Part model, mm, in its own coordinate system. A direction names the side the tool comes from. Give positions to 0.01 mm unless a question says otherwise; leave off trailing zeros. Order: outer loops, then holes, each group sorted by start corner. A loop starts at its lowest first (then second) coordinate and runs counter-clockwise, first axis right, second up. Notation, with made-up numbers: (3.25, -24.75) -> (24.25, -24.75) arc R21 cw to (24.25, 1.25) -> close; hole circle Ø1 at (38.25, 37). An arc over 180 degrees is marked (long way). Write item = value, one per line. Start each with the question number.
Item 1: Flat gauge pins, fed straight in: P1, Ø5, axis at y = -23.5, z = 1.5, coming from the -X side; P2, Ø1.5, axis at x = 15.5, z = 6, coming from the -Y side; P3, Ø1, axis at x = -35, z = 6.5, coming from the +Y side. Where does each tip first touch, or does it go through?
Item 2: Band-saw the part on A-A on x = 0. Write the cut outline in (y, z).
Item 3: Band-saw the part on B-B on y = 0. Write the cut outline in (x, z), plus the area to 3 significant figures.
Item 4: Tool access for faces 1 (the face through (22, -41, 0)), 2 (the face through (48, -11, 1.5)): list every direction of +Z, -Z, +X, -X, +Y, -Y with a clear straight run to the whole face (end or side of a thin tool).
Item 5: Pull direction X, two halves, no side cores. Call faces 3 (the face through (11, -47, 8.5)), 4 (the face through (-38.69, -29.66, 4.95)), 5 (the face through (-36.107, -27.686, 0.76)), 6 (the face through (-35.083, 32.17, 5.965)): +X half, -X half, draft (parallel to the pull), parting line (faces both ways), or undercut.
Item 6: Drill centre lines: line 1 along Y through (x, z) = (0, 1.05); line 2 along Y through (x, z) = (0, 7.45); line 3 along Z through (x, y) = (-28.5, 40.5). Where is each one in solid material? Low to high.
Item 7: Band-saw the part on C-C on z = 5.25. Write the cut outline in (x, y), plus the area to 3 significant figures.
```python
from build123d import *

# Parameters (mm, degrees)
F0_R     = 50
F1_DEPTH = 1.5
F2_R     = 48.75
F2_R_2   = 47.6
F3_DEPTH = 7
F4_R     = 45.5
F5_DEPTH = 25
F6_W     = 4.2
F6_H     = 2.5
F7_DEPTH = 150.9
F8_R     = 2


with BuildPart() as f1:
    # F0 (on Top) → F1 (new body)
    with BuildSketch(Plane.XY):
        Circle(F0_R)
    extrude(amount=F1_DEPTH)

    # F2 (on face) → F3 (join)
    with BuildSketch(Plane.XY.offset(1.5)):
        Circle(F2_R)
        Circle(F2_R_2, mode=Mode.SUBTRACT)
    extrude(amount=F3_DEPTH)

    # F4 (on face) → F5 (cut)
    with BuildSketch(Plane.XY.offset(1.5)):
        Circle(F4_R)
    extrude(amount=-F5_DEPTH, mode=Mode.SUBTRACT)

    # F6 (on Front) → F7 (cut)
    with BuildSketch(Plane.XZ):
        with Locations((0, 5.25)):
            Rectangle(F6_W, F6_H)
    extrude(amount=F7_DEPTH, mode=Mode.SUBTRACT)

    # F8
    f8_edges = [f1.edges().sort_by_distance(p)[0] for p in [
        (-47.6, 0, 1.5),
    ]]
    fillet(f8_edges, radius=F8_R)


solid = f1.part
```
Values found:
q1.P1 = -45.38
q1.P2 = -46.47
q1.P3 = 34.44
q2.outline = (-50, 0) -> (-45.5, 0) -> (-45.5, 1.5) -> (-45.6, 1.5) arc R2 cw to (-47.6, 3.5) -> (-47.6, 4) -> (-48.75, 4) -> (-48.75, 1.5) -> (-50, 1.5) -> close; (-48.75, 6.5) -> (-47.6, 6.5) -> (-47.6, 8.5) -> (-48.75, 8.5) -> close; (45.5, 0) -> (50, 0) -> (50, 1.5) -> (48.75, 1.5) -> (48.75, 8.5) -> (47.6, 8.5) -> (47.6, 3.5) arc R2 cw to (45.6, 1.5) -> (45.5, 1.5) -> close
q3.outline = (-50, 0) -> (-45.5, 0) -> (-45.5, 1.5) -> (-45.6, 1.5) arc R2 cw to (-47.6, 3.5) -> (-47.6, 8.5) -> (-48.75, 8.5) -> (-48.75, 1.5) -> (-50, 1.5) -> close; (45.5, 0) -> (50, 0) -> (50, 1.5) -> (48.75, 1.5) -> (48.75, 8.5) -> (47.6, 8.5) -> (47.6, 3.5) arc R2 cw to (45.6, 1.5) -> (45.5, 1.5) -> close
q3.area = 31.3 mm^2
q4.face_1 = -Z, +X, -X, +Y, -Y
q4.face_2 = +Z
q5.face_3 = draft
q5.face_4 = parting line
q5.face_5 = undercut
q5.face_6 = undercut
q6.line_1 = -50 to -45.5, 45.5 to 50
q6.line_2 = -48.75 to -47.6, 47.6 to 48.75
q6.line_3 = 0 to 1.5
q7.outline = (-2.1, -48.7) -> (-2.1, -47.55) arc R47.6 cw (long way) to (2.1, -47.55) -> (2.1, -48.7) arc R48.75 ccw (long way) to start
q7.area = 343 mm^2
